Could you check a few things on this model? Use its own coordinates, in mm. A direction names the side the tool comes from. Coordinates: 2 decimals unless noted, no trailing zeros. Order: outer loops, then holes, each group sorted by start corner. A loop starts at its lowest first (then second) coordinate and runs counter-clockwise, first axis right, second up. Notation, with made-up numbers: (77.25, -28.5) - (127.25, -28.5) arc R23 ccw to (127.25, 3.5) - close; hole circle Ø1 at (69, -34). An arc over 180 degrees is marked (long way). Answer as CSV lines item,"result". Start each with the question number.
1. For faces 1 (the face through (-2, -176, 114)), 2 (the face through (2, 175, 114)), which set-ups out of +Z, -Z, +X, -X, +Y, -Y let a thin tool reach every point of the face, with its end or its side?
2. Thinking about a two-plate mould opening in X: for faces 3 (the face through (-123, 14, 217)), 4 (the face through (-122, 14, 217)), 5 (the face through (123, -14, 217)), 6 (the face through (-2, 2, 232)), which applies, released by +X, released by -X, zero draft, split by the parting line, or undercut?
3. I want a section at A-A, the plane y = -110. List the corners of the cut face in (x, z) for me.
4. I need wall thicknesses on probe 1 along Y at (x, z) = (63, 151.5); probe 2 along Z at (x, y) = (113, 121); probe 3 along Z at (x, y) = (-79, 119.5). Which ranges of each line are inside material? Lowest first, please.
5. I want a section at B-B, the plane z = 132.5. List the corners of the cut face in (x, y) for me.
6. I want a section at C-C, the plane x = -65. List the corners of the cut face in (y, z) for me, and give its area (3 significant figures).
7. For pin 1 (1.1 mm diameter, centred on x = 122.5, z = 127, fed in from +Y); pin 2 (0.5 mm diameter, centred on y = -35.5, z = 0.5, fed in from +X); pin 3 (0.8 mm diameter, centred on x = 122.5, z = 83, fed in from -Y), each with a flat end and sliding along its axis, tell me the tip position at first contact or that it passes through.
from build123d import *

# Parameters (mm, degrees)
EXTRUDE_1_DEPTH     = 232
SKETCH_2_W          = 200
SKETCH_2_H          = 320
CUT_EXTRUDE_1_DEPTH = 500
EXTRUDE_START       = -1
EXTRUDE_1_2_DEPTH   = 1
SKETCH_4_W          = 214
SKETCH_4_H          = 320
EXTRUDE_2_DEPTH     = 1
FILLET_1_R          = 1
FILLET_2_R          = 2


with BuildPart() as part:
    # Эскиз1 → Extrude 1 (new body)
    with BuildSketch(Plane.XY):
        with BuildLine():
            Line((123, -173), (123, 173))
            ThreePointArc((123, 173), (122.121320344, 175.121320344), (120, 176))
            Line((120, 176), (-120, 176))
            ThreePointArc((-120, 176), (-122.121320344, 175.121320344), (-123, 173))
            Line((-123, 173), (-123, -173))
            ThreePointArc((-123, -173), (-122.121320344, -175.121320344), (-120, -176))
            Line((-120, -176), (120, -176))
            ThreePointArc((120, -176), (122.121320344, -175.121320344), (123, -173))
        make_face()
        with BuildLine():
            Line((122, -173), (122, 173))
            ThreePointArc((122, 173), (121.414213562, 174.414213562), (120, 175))
            Line((120, 175), (-120, 175))
            ThreePointArc((-120, 175), (-121.414213562, 174.414213562), (-122, 173))
            Line((-122, 173), (-122, -173))
            ThreePointArc((-122, -173), (-121.414213562, -174.414213562), (-120, -175))
            Line((-120, -175), (120, -175))
            ThreePointArc((120, -175), (121.414213562, -174.414213562), (122, -173))
        make_face(mode=Mode.SUBTRACT)
    extrude(amount=EXTRUDE_1_DEPTH)

    # Эскиз2 → Вырез-Вытянуть1 (cut)
    with BuildSketch(Plane(origin=(123, 0, 0), x_dir=(0, 0, -1), z_dir=(1, 0, 0))):
        with Locations((-116, 0)):
            Rectangle(SKETCH_2_W, SKETCH_2_H)
    extrude(amount=-CUT_EXTRUDE_1_DEPTH, mode=Mode.SUBTRACT)

    # Эскиз3 → Extrude 1 2 (add)
    with BuildSketch(Plane.XY.offset(232).offset(EXTRUDE_START)):
        with BuildLine():
            Line((-123, 173), (-123, -173))
            ThreePointArc((-123, -173), (-122.121320344, -175.121320344), (-120, -176))
            Line((-120, -176), (120, -176))
            ThreePointArc((120, -176), (122.121320344, -175.121320344), (123, -173))
            Line((123, -173), (123, 173))
            ThreePointArc((123, 173), (122.121320344, 175.121320344), (120, 176))
            Line((120, 176), (-120, 176))
            ThreePointArc((-120, 176), (-122.121320344, 175.121320344), (-123, 173))
        make_face()
    extrude(amount=EXTRUDE_1_2_DEPTH)

    # Эскиз4 → Вытянуть2 (add)
    with BuildSketch(Plane(origin=(0, 0, 0), x_dir=(-1, 0, 0), z_dir=(0, 0, -1))):
        with BuildLine():
            Line((120, 176), (-120, 176))
            ThreePointArc((-120, 176), (-122.121320344, 175.121320344), (-123, 173))
            Line((-123, 173), (-123, -173))
            ThreePointArc((-123, -173), (-122.121320344, -175.121320344), (-120, -176))
            Line((-120, -176), (120, -176))
            ThreePointArc((120, -176), (122.121320344, -175.121320344), (123, -173))
            Line((123, -173), (123, 173))
            ThreePointArc((123, 173), (122.121320344, 175.121320344), (120, 176))
        make_face()
        Rectangle(SKETCH_4_W, SKETCH_4_H, mode=Mode.SUBTRACT)
    extrude(amount=-EXTRUDE_2_DEPTH)

    # Скругление1
    fillet_1_edges = [part.edges().sort_by_distance(p)[0] for p in [
        (-122, 0, 1),
        (-121.414213562, 174.414213562, 1),
        (0, 175, 1),
        (121.414213562, 174.414213562, 1),
        (122, 0, 1),
        (121.414213562, -174.414213562, 1),
        (0, -175, 1),
        (-121.414213562, -174.414213562, 1),
        (0, 175, 231),
        (-121.414213562, 174.414213562, 231),
        (-122, 0, 231),
        (-121.414213562, -174.414213562, 231),
        (0, -175, 231),
        (121.414213562, -174.414213562, 231),
        (122, 0, 231),
        (121.414213562, 174.414213562, 231),
    ]]
    fillet(fillet_1_edges, radius=FILLET_1_R)

    # Скругление2
    fillet_2_edges = [part.edges().sort_by_distance(p)[0] for p in [
        (-122.121320344, -175.121320344, 232),
        (0, -176, 232),
        (122.121320344, -175.121320344, 232),
        (123, 0, 232),
        (122.121320344, 175.121320344, 232),
        (0, 176, 232),
        (-122.121320344, 175.121320344, 232),
        (0, 176, 0),
        (122.121320344, 175.121320344, 0),
        (123, 0, 0),
        (122.121320344, -175.121320344, 0),
        (0, -176, 0),
        (-122.121320344, -175.121320344, 0),
        (-123, 0, 0),
        (-122.121320344, 175.121320344, 0),
        (-123, 0, 232),
    ]]
    fillet(fillet_2_edges, radius=FILLET_2_R)


solid = part.part
Solved:
1,face 1,"+Z, -Z, +X, -X, -Y"
1,face 2,"none"
2,face 3,"released by -X"
2,face 4,"undercut"
2,face 5,"released by +X"
2,face 6,"zero draft"
3,outline,"(-123, 2) arc R2 ccw to (-121, 0) - (-107, 0) - (-107, 1) - (-121, 1) arc R1 cw to (-122, 2) - (-122, 16) - (-123, 16) - close; (-123, 216) - (-122, 216) - (-122, 230) arc R1 cw to (-121, 231) - (121, 231) arc R1 cw to (122, 230) - (122, 216) - (123, 216) - (123, 230) arc R2 ccw to (121, 232) - (-121, 232) arc R2 ccw to (-123, 230) - close; (107, 0) - (121, 0) arc R2 ccw to (123, 2) - (123, 16) - (122, 16) - (122, 2) arc R1 cw to (121, 1) - (107, 1) - close"
4,probe 1,"y = -176 to -175, 175 to 176"
4,probe 2,"z = 0 to 1, 231 to 232"
4,probe 3,"z = 231 to 232"
5,outline,"(-123, -173) arc R3 ccw to (-120, -176) - (120, -176) arc R3 ccw to (123, -173) - (123, -160) - (122, -160) - (122, -173) arc R2 cw to (120, -175) - (-120, -175) arc R2 cw to (-122, -173) - (-122, -160) - (-123, -160) - close; (-123, 160) - (-122, 160) - (-122, 173) arc R2 cw to (-120, 175) - (120, 175) arc R2 cw to (122, 173) - (122, 160) - (123, 160) - (123, 173) arc R3 ccw to (120, 176) - (-120, 176) arc R3 ccw to (-123, 173) - close"
6,outline,"(-176, 2) arc R2 ccw to (-174, 0) - (-160, 0) - (-160, 1) - (-174, 1) arc R1 cw to (-175, 2) - (-175, 230) arc R1 cw to (-174, 231) - (174, 231) arc R1 cw to (175, 230) - (175, 2) arc R1 cw to (174, 1) - (160, 1) - (160, 0) - (174, 0) arc R2 ccw to (176, 2) - (176, 230) arc R2 ccw to (174, 232) - (-174, 232) arc R2 ccw to (-176, 230) - close"
6,area,"841 mm2"
7,pin 1,"stops at y = 175.28"
7,pin 2,"stops at x = 122.56"
7,pin 3,"stops at y = -175.14"
